Input: part model. Units: mm. Frame: model coordinates. Round coordinates to 2 decimals unless told otherwise and drop trailing zeros. Put each result on its own line as item: value. Start each with the question number.
1) Line query: probe 1 along Z at (x, y) = (66.5, 1.75); probe 2 along Y at (x, z) = (68.5, 48); probe 3 along Y at (x, z) = (57, 2.4). Output: solid intervals per line, ascending.
2) Pin query (flat end, axial travel): pin 1 (2 mm diameter, centred on x = 72.5, z = 71, fed in from +Y); pin 2 (6 mm diameter, centred on x = 44.5, z = 26.5, fed in from +Y); pin 3 (3.5 mm diameter, centred on y = 2.5, z = 43.5, fed in from -X). Return the tip coordinate at first contact, or that it passes through.
3) Section A-A on z = 24. State how many separate pieces and enclosed holes the cut face has, plus the area to 3 significant figures.
from build123d import *
from OCP.BRepFilletAPI import BRepFilletAPI_MakeChamfer

# Parameters (mm, degrees)
SKETCH4_R          = 2.6
SKETCH4_R_2        = 3.1
CUT_EXTRUDE1_DEPTH = 5.2
SKETCH5_W          = 9.9
SKETCH5_H          = 6
SKETCH5_W_2        = 9.5
CUT_EXTRUDE2_DEPTH = 70
FILLET3_R          = 2
CHAMFER1_SIZE      = 1
CHAMFER1_SIZE2     = 1.191753593
CUT_EXTRUDE3_DEPTH = 90.2
FILLET4_R          = 0.2
FILLET5_R          = 0.5
CHAMFER2_SIZE      = 1


with BuildPart() as part:
    # Sketch1 → Loft1 section 0
    with BuildSketch(Plane.XY):
        with BuildLine():
            add(Edge.make_bspline(
                [(115, 0), (114.999913382, 0.00327866), (114.222934603, -0.004567066), (113.418136575, 0.000318408), (111.44543546, 0.018706002), (108.999380922, 0.080565277), (105.780115155, 0.203144323), (101.978037922, 0.467320429), (97.63148646, 0.880990765), (92.843812566, 1.427373326), (87.693014802, 2.062174327), (82.26127365, 2.794917392), (76.628898252, 3.582200475), (70.875421432, 4.408274793), (65.069516957, 5.204495648), (59.272555938, 5.964988559), (53.535411353, 6.612069385), (47.902032041, 7.147901639), (42.420677472, 7.538059951), (37.125743857, 7.784294524), (32.060080889, 7.863888962), (27.260899934, 7.799703202), (22.764274035, 7.585443948), (18.606628598, 7.224009749), (14.819582747, 6.717397261), (11.43119341, 6.102885155), (8.463318021, 5.359495242), (5.929953708, 4.523167874), (3.840235227, 3.611431652), (2.203139301, 2.680524392), (0.997143498, 1.719388226), (0.306055902, 0.84473605), (-0.153897847, -0.016785493), (0.441131195, -0.783771302), (1.630250645, -0.976182526), (3.345026164, -1.247099953), (5.741349663, -1.385446358), (8.741002332, -1.531007587), (12.32356917, -1.613427576), (16.426146399, -1.711956772), (20.996614723, -1.764001286), (25.979915364, -1.804105207), (31.316658928, -1.826220598), (36.950031377, -1.811871436), (42.810070502, -1.783755804), (48.833365319, -1.730024981), (54.950109545, -1.67348399), (61.093513049, -1.595166549), (67.193299365, -1.488121719), (73.176935484, -1.397778739), (78.980025922, -1.271232402), (84.533413271, -1.152999753), (89.776869938, -1.037364871), (94.647010434, -0.905039683), (99.089599698, -0.778312882), (103.055602703, -0.646322839), (106.488295637, -0.529569147), (109.391284428, -0.370730171), (111.629000068, -0.244208643), (113.467096811, -0.099576309), (114.237158295, -0.036931621), (115.000086752, -0.003283716), (115, 0)],
                knots=[0, 0, 0, 0, 0.001545172, 0.006223608, 0.014035782, 0.024855049, 0.038644124, 0.055163693, 0.074045466, 0.094820373, 0.117222732, 0.140866367, 0.165395395, 0.190452399, 0.215710088, 0.240854358, 0.265734023, 0.290048364, 0.313714428, 0.336486101, 0.358292895, 0.378940292, 0.398278007, 0.416246563, 0.432660408, 0.447459903, 0.460566131, 0.472021733, 0.481783695, 0.489844359, 0.496307136, 0.50126117, 0.504695153, 0.507385543, 0.512190444, 0.519692984, 0.529980259, 0.542956454, 0.558414131, 0.576101982, 0.595804604, 0.61726601, 0.64027206, 0.66452271, 0.689803764, 0.7157292, 0.742084221, 0.768568973, 0.794840399, 0.820639753, 0.845625339, 0.869581038, 0.892163588, 0.913159587, 0.932310678, 0.94940252, 0.964220925, 0.976641917, 0.986532119, 0.993892864, 0.998452446, 1, 1, 1, 1], degree=3))
        make_face()
    # Sketch2 → Loft1 section 1
    with BuildSketch(Plane.XY.offset(110)):
        with BuildLine():
            add(Edge.make_bspline(
                [(110, 0), (110.000464145, 0.002638021), (109.253557002, -0.006421882), (108.485306247, 0.00202473), (106.599515685, 0.014018922), (104.259903283, 0.071192731), (101.178986874, 0.200889618), (97.542661477, 0.451950761), (93.384633146, 0.843539364), (88.805204424, 1.362015696), (83.880374164, 1.978555721), (78.68657223, 2.677523385), (73.299477431, 3.430735281), (67.795235431, 4.215247142), (62.241233075, 4.984660857), (56.695525551, 5.697469803), (51.207787306, 6.322755672), (45.821489693, 6.833626486), (40.577824462, 7.211562863), (35.514283248, 7.444282984), (30.668486135, 7.527509184), (26.076763803, 7.463490784), (21.77566696, 7.255221358), (17.798933432, 6.909184212), (14.177047879, 6.430194992), (10.935139134, 5.831964767), (8.094704102, 5.122344568), (5.670248347, 4.327180111), (3.669790047, 3.460558372), (2.10909167, 2.56151381), (0.952680778, 1.647952784), (0.292493833, 0.810328248), (-0.144477468, -0.013443729), (0.421457768, -0.751792674), (1.561430619, -0.927732015), (3.196411713, -1.199647616), (5.489901797, -1.325203312), (8.359384575, -1.457341268), (11.786506209, -1.55318322), (15.712038629, -1.632817261), (20.085890157, -1.693490267), (24.85332264, -1.730533844), (29.958495668, -1.745317698), (35.344133299, -1.736641885), (40.949025669, -1.70754651), (46.710109342, -1.660092686), (52.562107594, -1.595708584), (58.438334584, -1.519615465), (64.272360823, -1.429130605), (69.997133878, -1.329443239), (75.548112692, -1.222377083), (80.861507128, -1.10840335), (85.876724326, -0.990587124), (90.536246874, -0.869398239), (94.784781842, -0.746694986), (98.577741113, -0.621781265), (101.858350076, -0.496229968), (104.635869759, -0.366297292), (106.773720091, -0.224338993), (108.53252638, -0.099668194), (109.269457647, -0.031974616), (109.999539654, -0.002616432), (110, 0)],
                knots=[0, 0, 0, 0, 0.001564721, 0.006239121, 0.014018617, 0.024861007, 0.038659987, 0.055174427, 0.074046407, 0.094837256, 0.117226118, 0.14085626, 0.165386109, 0.19045125, 0.215702393, 0.240866612, 0.265718976, 0.290051983, 0.313696202, 0.33648442, 0.358279861, 0.378929437, 0.398292398, 0.416235766, 0.432650472, 0.447455618, 0.460592079, 0.472030369, 0.48177877, 0.489853088, 0.496315276, 0.501246195, 0.504684904, 0.507403743, 0.512183233, 0.519672773, 0.529968131, 0.54294809, 0.558399818, 0.576099165, 0.595810572, 0.617282889, 0.64027984, 0.664535393, 0.689783385, 0.715732831, 0.742092653, 0.768566703, 0.794844175, 0.820638712, 0.845644257, 0.86958445, 0.892182833, 0.913177877, 0.932327829, 0.949410904, 0.964230176, 0.976629486, 0.986536787, 0.993881551, 0.998448084, 1, 1, 1, 1], degree=3))
        make_face()
    loft()

    # Sketch4 → Cut-Extrude1 (cut)
    with BuildSketch(Plane(origin=(0, 0, 0), x_dir=(-1, 0, 0), z_dir=(0, 0, -1))):
        with Locations((-10.5, 2)):
            Circle(SKETCH4_R)
        with Locations((-57, 2.1)):
            Circle(SKETCH4_R_2)
    extrude(amount=-CUT_EXTRUDE1_DEPTH, mode=Mode.SUBTRACT)

    # Sketch5 → Cut-Extrude2 (cut)
    with BuildSketch(Plane(origin=(0, 0, 0), x_dir=(-1, 0, 0), z_dir=(0, 0, -1))):
        with Locations((-21, 2.8)):
            Rectangle(SKETCH5_W, SKETCH5_H)
        with Locations((-46, 3)):
            Rectangle(SKETCH5_W_2, SKETCH5_H)
    extrude(amount=-CUT_EXTRUDE2_DEPTH, mode=Mode.SUBTRACT)

    # Fillet3
    fillet3_edges = [part.edges().sort_by_distance(p)[0] for p in [
        (16.05, 5.8, 35),
        (25.95, 5.8, 35),
        (41.25, 6, 35),
        (50.75, 6, 35),
    ]]
    fillet(fillet3_edges, radius=FILLET3_R)

    # Chamfer1: one chamfer whose edges measure the first distance from different faces: ONE call of the kernel's chamfer builder (chamfer() names one face for all edges)
    chamfer1_edges_1 = [part.edges().sort_by_distance(p)[0] for p in [
        (16.05, -0.2, 35),
    ]]
    chamfer1_side_1 = [part.faces().sort_by_distance(p)[0] for p in [
        (21, -0.2, 35),
    ]]
    chamfer1_edges_2 = [part.edges().sort_by_distance(p)[0] for p in [
        (25.95, -0.2, 35),
    ]]
    chamfer1_side_2 = [part.faces().sort_by_distance(p)[0] for p in [
        (25.95, 1.8, 35),
    ]]
    chamfer1_edges_3 = [part.edges().sort_by_distance(p)[0] for p in [
        (41.25, 0, 35),
    ]]
    chamfer1_side_3 = [part.faces().sort_by_distance(p)[0] for p in [
        (46, 0, 35),
    ]]
    chamfer1_edges_4 = [part.edges().sort_by_distance(p)[0] for p in [
        (50.75, 0, 35),
    ]]
    chamfer1_side_4 = [part.faces().sort_by_distance(p)[0] for p in [
        (50.75, 2, 35),
    ]]
    chamfer1 = BRepFilletAPI_MakeChamfer(part.part.solid().wrapped)
    for e in chamfer1_edges_1:
        chamfer1.Add(CHAMFER1_SIZE, CHAMFER1_SIZE2, e.wrapped, chamfer1_side_1[0].wrapped)  # the first distance lies on this face
    for e in chamfer1_edges_2:
        chamfer1.Add(CHAMFER1_SIZE, CHAMFER1_SIZE2, e.wrapped, chamfer1_side_2[0].wrapped)  # the first distance lies on this face
    for e in chamfer1_edges_3:
        chamfer1.Add(CHAMFER1_SIZE, CHAMFER1_SIZE2, e.wrapped, chamfer1_side_3[0].wrapped)  # the first distance lies on this face
    for e in chamfer1_edges_4:
        chamfer1.Add(CHAMFER1_SIZE, CHAMFER1_SIZE2, e.wrapped, chamfer1_side_4[0].wrapped)  # the first distance lies on this face
    add(Compound.cast(chamfer1.Shape()), mode=Mode.REPLACE)

    # Sketch6 → Cut-Extrude3 (cut)
    with BuildSketch(Plane(origin=(0, 0, 0), x_dir=(-1, 0, 0), z_dir=(0, 0, -1))):
        Polygon((-63.462295223, 3.793174257), (-63.462295223, 0.235158592), (-89.865630471, 0.235158592), align=None)
    extrude(amount=-CUT_EXTRUDE3_DEPTH, mode=Mode.SUBTRACT)

    # Fillet4
    fillet4_edges = [part.edges().sort_by_distance(p)[0] for p in [
        (89.865630471, 0.235158592, 45.1),
    ]]
    fillet(fillet4_edges, radius=FILLET4_R)

    # Fillet5
    fillet5_edges = [part.edges().sort_by_distance(p)[0] for p in [
        (63.462295223, 3.793174257, 45.1),
    ]]
    fillet(fillet5_edges, radius=FILLET5_R)

    # Chamfer2
    chamfer2_edges = [part.edges().sort_by_distance(p)[0] for p in [
        (63.462295223, 0.235158592, 45.1),
    ]]
    chamfer(chamfer2_edges, length=CHAMFER2_SIZE)


solid = part.part
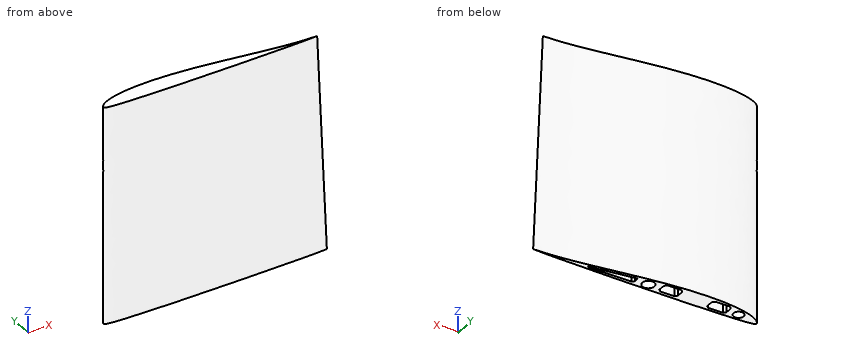
Geometry results:
1. probe 1: z = 90.2 to 110
1. probe 2: y = -1.42 to 0.24, 3.11 to 4.46
1. probe 3: y = -1.64 to -1, 5.2 to 6.2
2. pin 1: stops at y = 3.91
2. pin 2: stops at y = 7.47
2. pin 3: stops at x = 0.28
3. separate pieces: 1
3. enclosed holes: 3
3. area: 512 mm²
